Geometry check sheet. Reference: the model listing, model coordinates, mm. A direction names the side the tool comes from. Round coordinates to 2 decimals unless told otherwise and drop trailing zeros. Order: outer loops, then holes, each group sorted by start corner. A loop starts at its lowest first (then second) coordinate and runs counter-clockwise, first axis right, second up. Notation, with made-up numbers: (-11, -10) - (-5, -10) arc R26 cw to (-5, 25) - close; hole circle Ø10 at (-27, 34.25). An arc over 180 degrees is marked (long way). Answer as CSV lines item,"result". Start each with the question number.
Autodesk Inventor part; units mm, degrees
ref_plane "YZ Plane" through (0, 0, 0) normal (1, 0, 0) x (0, 1, 0)
ref_plane "XZ Plane" through (0, 0, 0) normal (0, 1, 0) x (-1, 0, 0)
ref_plane "XY Plane" through (0, 0, 0) normal (0, 0, 1) x (1, 0, 0)
sketch "Sketch3" plane through (0, 0, 0) normal (0, 1, 0) x (-1, 0, 0)
  line L0 (3, -20.5) -> (3, -14.5)
  line L1 (13, 20.5) -> (3, 20.5)
  line L2 (3, -20.5) -> (3, 20.5)
  line L3 (3, 20.5) -> (13, 20.5)
  line L4 (13, 20.5) -> (13, -20.5)
  line L5 (13, -20.5) -> (3, -20.5)
  line L6 (0, 0) -> (3, 0)
  line L7 (13, 14.5) -> (3, 14.5)
  line L8 (3, -14.5) -> (13, -14.5)
  line L9 (3, -14.5) -> (13, -14.5)
  line L10 (3, 14.5) -> (13, 14.5)
  circle A0 centre (8, -17.508) radius 1.425
  circle A1 centre (8, -17.508) radius 1.425
  circle A2 centre (8, 17.4854) radius 1.425
  circle A3 centre (8, 17.4854) radius 1.425
  point P0 (3, 20.5)
  dimension "d15" = 41
  dimension "d16" = 10
  dimension "d17" = 0
  dimension "d18" = 6
extrude "Extrusion1" add sketch "Sketch3" along normal blind 1
sketch "Sketch5" plane through (0, 0, 0) normal (0, -1, 0) x (1, 0, 0)
  line L0 (-3, 20.5) -> (-3, 14.5)
  line L1 (-13, -20.5) -> (-3, -20.5)
  line L2 (-3, 20.5) -> (-3, -20.5)
  line L3 (-3, -20.5) -> (-13, -20.5)
  line L4 (-13, -20.5) -> (-13, 20.5)
  line L5 (-13, 20.5) -> (-3, 20.5)
  line L6 (0, 0) -> (-3, 0)
  line L7 (-13, -14.5) -> (-3, -14.5)
  line L8 (-3, 14.5) -> (-13, 14.5)
  line L9 (-3, 14.5) -> (-13, 14.5)
  line L10 (-3, -14.5) -> (-13, -14.5)
  circle A0 centre (-8, 17.508) radius 1.425
  circle A1 centre (-8, 17.508) radius 1.425
  circle A2 centre (-8, -17.4854) radius 1.425
  circle A3 centre (-8, -17.4854) radius 1.425
  circle A4 centre (0, 0) radius 11
  circle A5 centre (0, 0) radius 13
  point P0 (3, 20.5)
  point P1 (3, -14.5)
  point P2 (-3, 12.6491)
  point P3 (-3, 10.583)
  point P4 (-3, -10.583)
  point P5 (-3, -12.6491)
  dimension "d27" = 41
  dimension "d28" = 10
  dimension "d29" = 0
  dimension "d30" = 6
  dimension "d31" = 22
  dimension "d32" = 26
extrude "Extrusion2" add sketch "Sketch5" against normal blind 9 contours A5 L2 A4 | L2 A4 A5
sketch "Sketch6" plane through (0, 9, 0) normal (0, 1, 0) x (1, 0, 0)
  circle A0 centre (0, 0) radius 11
extrude "Extrusion3" cut sketch "Sketch6" against normal through all
properties part number "Ball_Bearing_Holder"
1. Go/stop test with flat-tipped pins: pin 1 Ø4.5 at (x, z) = (-8, -17.508) entering from +Y; pin 2 Ø3 at (x, z) = (-8.5, 11.5) entering from +Y; pin 3 Ø2 at (y, z) = (8, -11) entering from -X; pin 4 Ø4 at (x, y) = (-1, 3) entering from +Z. Record where each tip stops, or that it passes through.
2. Section check B-B on z = 2. Record the boundary of the cut face in (x, y), plus the area to 3 significant figures.
3. Draft check along X on faces 1 (the face through (-7.814, 0.493, 16.073)), 2 (the face through (-13, 0.5, 0.3)), 3 (the face through (-9, 1, 15)). Enter one of: released by +X, released by -X, zero draft, split by the parting line, or undercut.
4. Section check D-D on x = -8. Record the boundary of the cut face in (y, z).
5. Access from +Z, -Z, +X, -X, +Y, -Y to the whole of each face (thin tool, end or side, straight path). Record for faces 4 (the face through (12, 4, -5)), 5 (the face through (-8.1, 0.5, -20.5)), 6 (the face through (-9, 1, -15)).
6. Section check C-C on y = 8.25. Record the boundary of the cut face in (x, z).
7. Thickness scan on probe 1 along X at (y, z) = (3, 0); probe 2 along Z at (x, y) = (-8, 0.55). Record the ranges inside material, lowest first.
8. Section check A-A on x = 0. Record the boundary of the cut face in (y, z).
Numbers:
1,pin 1,"stops at y = 1"
1,pin 2,"stops at y = 9"
1,pin 3,"stops at x = -8.31"
1,pin 4,"stops at z = 13"
2,outline,"(-13, 0) - (-10.82, 0) - (-10.82, 9) - (-12.85, 9) - (-12.85, 1) - (-13, 1) - close; (10.82, 0) - (12.85, 0) - (12.85, 9) - (10.82, 9) - close"
2,area,"36.7 mm2"
3,face 1,"undercut"
3,face 2,"released by -X"
3,face 3,"zero draft"
4,outline,"(0, -20.5) - (1, -20.5) - (1, -18.93) - (0, -18.93) - close; (0, -16.08) - (1, -16.08) - (1, -10.25) - (9, -10.25) - (9, -7.55) - (0, -7.55) - close; (0, 7.55) - (9, 7.55) - (9, 10.25) - (1, 10.25) - (1, 16.06) - (0, 16.06) - close; (0, 18.91) - (1, 18.91) - (1, 20.5) - (0, 20.5) - close"
5,face 4,"+Y"
5,face 5,"-Z, +X, -X, +Y, -Y"
5,face 6,"-Z, -X, +Y"
6,outline,"circle Ø26 at (0, 0); hole circle Ø22 at (0, 0)"
7,probe 1,"x = -13 to -11, 11 to 13"
7,probe 2,"z = -20.5 to -18.93, -16.08 to -7.55, 7.55 to 16.06, 18.91 to 20.5"
8,outline,"(0, -13) - (9, -13) - (9, -11) - (0, -11) - close; (0, 11) - (9, 11) - (9, 13) - (0, 13) - close"
